Source: CAD feature listing. Evaluate the final solid. Frame: model axes, mm. A direction names the side the tool comes from. Round coordinates to 2 decimals unless told otherwise and drop trailing zeros. Order: outer loops, then holes, each group sorted by start corner. A loop starts at its lowest first (then second) coordinate and runs counter-clockwise, first axis right, second up. Notation, with made-up numbers: (16.25, 3.25) -> (25.25, 3.25) arc R33 cw to (25.25, 42.25) -> close; hole circle Ø10 at (-11.5, 0). An arc over 180 degrees is marked (long way). Write item = value, one per line. Start each with the question number.
(1) Contact query for flat-ended pins moving along their axis: pin 1 Ø5 at (x, z) = (-13, 4) entering from +Y; pin 2 Ø1 at (y, z) = (-12.5, 3.5) entering from -X; pin 3 Ø5 at (x, z) = (-8.5, 4.5) entering from +Y. Output: stop coordinate, or through.
(2) Cut plane B-B on x = 0. Return the cut outline in (y, z), then the cut area to 3 significant figures.
(3) Cut plane A-A on z = 4.25. Return the cut outline in (x, y), then the cut area to 3 significant figures.
(4) Cut plane C-C on z = 1.25. Return the cut outline in (x, y).
(5) Draft query along X for faces 3 (the face through (-4.336, -19.524, 6.549)), 4 (the face through (0, 0, 10)), 5 (the face through (-0.5, 0, 5)). Return one class per face: released by +X, released by -X, zero draft, split by the parting line, or undercut.
(6) Reachability of faces 1 (the face through (0, 0, -2)), 2 (the face through (-1, 0, 0)) from +Z, -Z, +X, -X, +Y, -Y: full face, straight path, thin tool, end or side. Return the list, or none.
(7) Ray query, line 1 (Y direction, x = 1.5, z = 8.5); line 2 (Y direction, x = -5.5, z = 0.25); line 3 (X direction, y = 7.5, z = -1.25). Return the intervals inside material, ascending.
from build123d import *

# Parameters (mm, degrees)
F0_R     = 20
F1_DEPTH = 10
F2_DEPTH = 2
F3_R     = 5


with BuildPart() as f1:
    # F0 (on Top) → F1 (new body)
    with BuildSketch(Plane.XY):
        Circle(F0_R)
        with BuildLine():
            ThreePointArc((0.5, 1.936492), (1.581139, 1.224745), (2, 0))
            ThreePointArc((2, 0), (1.581139, -1.224745), (0.5, -1.936492))
            ThreePointArc((0.5, -1.936492), (0, -2), (-0.5, -1.936492))
            ThreePointArc((-0.5, -1.936492), (-2, 0), (-0.5, 1.936492))
            ThreePointArc((-0.5, 1.936492), (0, 2), (0.5, 1.936492))
        make_face(mode=Mode.SUBTRACT)
        with BuildLine():
            Line((0.5, 0), (0.5, 1.936492))
            ThreePointArc((0.5, 1.936492), (0, 2), (-0.5, 1.936492))
            Line((-0.5, 1.936492), (-0.5, 0))
            Line((-0.5, 0), (-0.5, -1.936492))
            ThreePointArc((-0.5, -1.936492), (0, -2), (0.5, -1.936492))
            Line((0.5, -1.936492), (0.5, 0))
        make_face()
    extrude(amount=F1_DEPTH)

    # F0 (on Top) → F2 (join)
    with BuildSketch(Plane.XY):
        Circle(F0_R)
        with BuildLine():
            ThreePointArc((0.5, 1.936492), (1.581139, 1.224745), (2, 0))
            ThreePointArc((2, 0), (1.581139, -1.224745), (0.5, -1.936492))
            ThreePointArc((0.5, -1.936492), (0, -2), (-0.5, -1.936492))
            ThreePointArc((-0.5, -1.936492), (-2, 0), (-0.5, 1.936492))
            ThreePointArc((-0.5, 1.936492), (0, 2), (0.5, 1.936492))
        make_face(mode=Mode.SUBTRACT)
        with BuildLine():
            ThreePointArc((0.5, -1.936492), (1.581139, -1.224745), (2, 0))
            ThreePointArc((2, 0), (1.581139, 1.224745), (0.5, 1.936492))
            Line((0.5, 1.936492), (0.5, 0))
            Line((0.5, 0), (0.5, -1.936492))
        make_face()
        with BuildLine():
            Line((-0.5, 0), (-0.5, 1.936492))
            ThreePointArc((-0.5, 1.936492), (-2, 0), (-0.5, -1.936492))
            Line((-0.5, -1.936492), (-0.5, 0))
        make_face()
        with BuildLine():
            Line((0.5, 0), (0.5, 1.936492))
            ThreePointArc((0.5, 1.936492), (0, 2), (-0.5, 1.936492))
            Line((-0.5, 1.936492), (-0.5, 0))
            Line((-0.5, 0), (-0.5, -1.936492))
            ThreePointArc((-0.5, -1.936492), (0, -2), (0.5, -1.936492))
            Line((0.5, -1.936492), (0.5, 0))
        make_face()
    extrude(amount=-F2_DEPTH)

    # F3
    f3_edges = [f1.edges().sort_by_distance(p)[0] for p in [
        (-20, 0, -2),
    ]]
    fillet(f3_edges, radius=F3_R)


solid = f1.part
Evaluation:
q1.pin_1 = 17.02
q1.pin_2 = -16
q1.pin_3 = 19.08
q2.outline = (-20, 3) arc R5 ccw to (-15, -2) -> (15, -2) arc R5 ccw to (20, 3) -> (20, 10) -> (-20, 10) -> close
q2.area = 469 mm^2
q3.outline = circle Ø40 at (0, 0); hole (-0.5, -1.94) -> (-0.5, 1.94) arc R2 ccw to start; hole (0.5, -1.94) arc R2 ccw to (0.5, 1.94) -> close
q3.area = 1,250 mm^2
q4.outline = circle Ø39.37 at (0, 0); hole (-0.5, -1.94) -> (-0.5, 1.94) arc R2 ccw to start; hole (0.5, -1.94) arc R2 ccw to (0.5, 1.94) -> close
q5.face_3 = split by the parting line
q5.face_4 = zero draft
q5.face_5 = undercut
q6.face_1 = -Z, +X, -X, +Y, -Y
q6.face_2 = +Z
q7.line_1 = -19.94 to -1.32, 1.32 to 19.94
q7.line_2 = -18.37 to 18.37
q7.line_3 = -15.96 to 15.96
